Geometry: see drawing. Coordinates: mm, zero at the bounding-box minimum. Give positions to 0.01 mm unless a question says otherwise; leave off trailing zeros. Order: outer loops, then holes, each group sorted by start corner. A loop starts at its lowest first (then second) coordinate and runs counter-clockwise, first axis right, second up. Notation, with made-up numbers: M -11.75,11.5 L 33.25,11.5 A18 cw 33.25,43.5 Z; hole C 26,-38 d3. An arc over 180 degrees is marked long. Return JSON: item names as keys, results as strings.
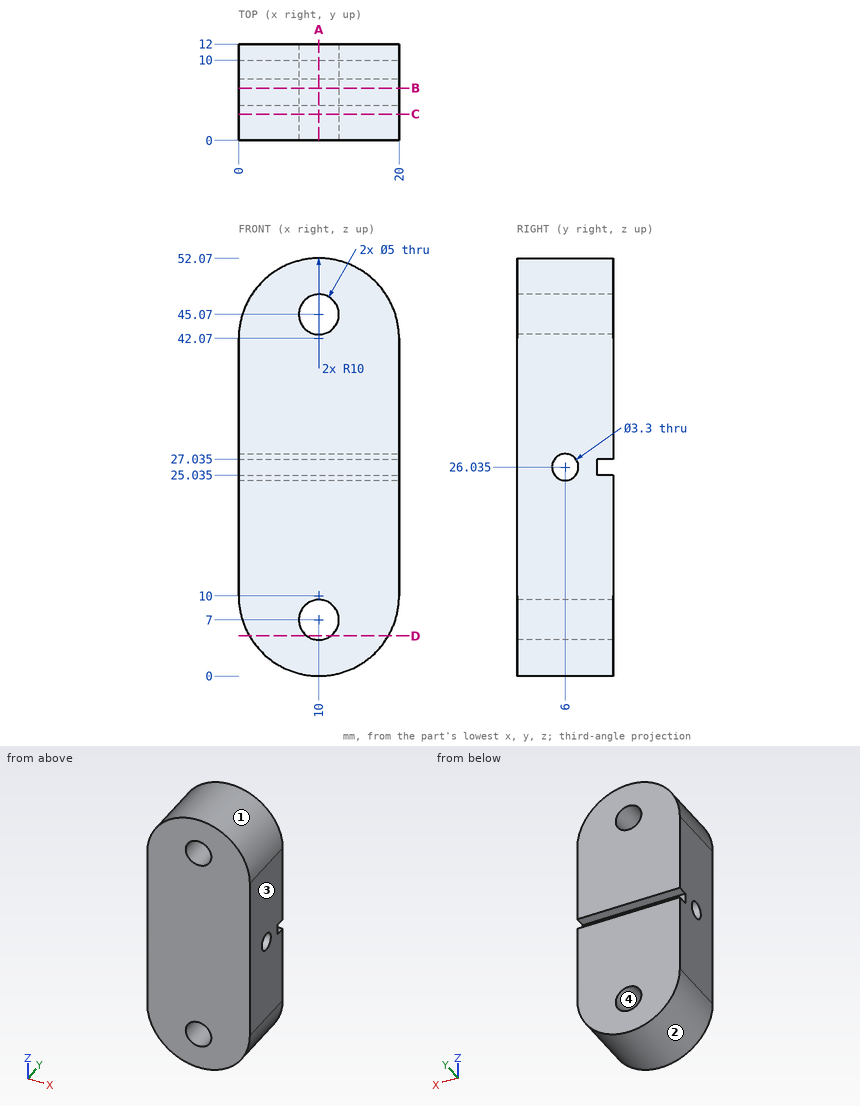
1. Section query C-C (y = 3.25). Return loops of the section in (x, z), then the cut area to 3 significant figures.
Evaluation:
{"outline": "M 0,10 A10 ccw 20,10 L 20,42.07 A10 ccw 0,42.07 Z; hole C 10,7 d5; hole C 10,45.07 d5", "area": "916 mm^2"}
2. First-contact query: pin 1 (1.6 mm diameter, centred on x = 9, y = 11, fed in from -Z); pin 2 (0.6 mm diameter, centred on x = 9, z = 25.5, fed in from +Y); pin 3 (5 mm diameter, centred on x = 14, y = 9.5, fed in from -Z). Flat tips, straight axial feed; report the tip coordinate or a pass-through.
Evaluation:
{"pin 1": "stops at z = 0", "pin 2": "stops at y = 10", "pin 3": "stops at z = 0.11"}
3. Section query A-A (x = 10). Return loops of the section in (y, z) (3 decimals), then the cut area to 3 significant figures.
Evaluation:
{"outline": "M 0,0 L 12,0 L 12,4.5 L 0,4.5 Z; M 0,9.5 L 12,9.5 L 12,25.035 L 10,25.035 L 10,27.035 L 12,27.035 L 12,42.57 L 0,42.57 Z; M 0,47.57 L 12,47.57 L 12,52.07 L 0,52.07 Z; hole C 6,26.035 d3.3", "area": "492 mm^2"}
4. Section query D-D (z = 5). Return loops of the section in (x, y), then the cut area to 3 significant figures.
Evaluation:
{"outline": "M 1.34,0 L 8.5,0 L 8.5,12 L 1.34,12 Z; M 11.5,0 L 18.66,0 L 18.66,12 L 11.5,12 Z", "area": "172 mm^2"}
5. Draft query along Z for the marked faces 1, 2, 3 and 4. Return one class per face: pulls with the +Z half, pulls with the -Z half, needs draft (parallel to the pull), parting line crosses it, or undercut.
Evaluation:
{"face 1": "pulls with the +Z half", "face 2": "pulls with the -Z half", "face 3": "needs draft", "face 4": "undercut"}
6. Section query B-B (y = 6.5). Return loops of the section in (x, z).
Evaluation:
{"outline": "M 0,10 A10 ccw 20,10 L 20,24.46 L 0,24.46 Z; M 0,27.61 L 20,27.61 L 20,42.07 A10 ccw 0,42.07 Z; hole C 10,7 d5; hole C 10,45.07 d5"}
7. Ray query, probe 1 along Z at (x, y) = (10, 3.5); probe 2 along Z at (x, y) = (12, 5); probe 3 along Z at (x, y) = (10, 5). Return the intervals inside material, ascending.
Evaluation:
{"probe 1": "z = 0 to 4.5, 9.5 to 42.57, 47.57 to 52.07", "probe 2": "z = 0.2 to 5.5, 8.5 to 24.72, 27.35 to 43.57, 46.57 to 51.87", "probe 3": "z = 0 to 4.5, 9.5 to 24.72, 27.35 to 42.57, 47.57 to 52.07"}
